Input: part model. Units: mm. Frame: model coordinates. A direction names the side the tool comes from. Give positions to 0.01 mm unless a question says otherwise; leave off trailing zeros. Write each loop counter-clockwise with the first axis right and the second up, starting at its lowest first coordinate (ties: lowest second). Pieces come first, ordered by that corner, then holes.
```python
from build123d import *

# Parameters (mm, degrees)
SKETCH1_R           = 10.16
BOSS_EXTRUDE1_DEPTH = 66.04
SKETCH2_R           = 12.7
BOSS_EXTRUDE2_DEPTH = 2.54
BOSS_EXTRUDE3_START = -2.54
SKETCH3_R           = 12.7
BOSS_EXTRUDE3_DEPTH = 2.54


with BuildPart() as part:
    # Sketch1 → Boss-Extrude1 (new, symmetric)
    with BuildSketch(Plane(origin=(0, 0, 0), x_dir=(1, 0, 0), z_dir=(0, 1, 0))):
        with Locations(Location((0, 0, 0), (0, 0, 270))):
            Circle(SKETCH1_R)
    extrude(amount=BOSS_EXTRUDE1_DEPTH, both=True)

    # Sketch2 → Boss-Extrude2 (add)
    with BuildSketch(Plane(origin=(0, 66.04, 0), x_dir=(1, 0, 0), z_dir=(0, 1, 0))):
        with Locations(Location((0, 0, 0), (0, 0, 270))):
            Circle(SKETCH2_R)
    extrude(amount=-BOSS_EXTRUDE2_DEPTH)

    # Sketch3 → Boss-Extrude3 (add)
    with BuildSketch(Plane.XZ.offset(66.04).offset(BOSS_EXTRUDE3_START)):
        with Locations(Location((0, 0, 0), (0, 0, 90))):
            Circle(SKETCH3_R)
    extrude(amount=BOSS_EXTRUDE3_DEPTH)


solid = part.part
```
Item 1: Mould query, pull axis Y, two halves, no side actions, for faces 3 (the cylindrical face through (7.7, -64.8, -10.1)), 4 (the flat face through (0, -66.04, 0)), 5 (the flat face through (0, 66.04, 0)), 6 (the flat face through (9, 63.5, -6)). Classes: +Y half, -Y half, draft (parallel to the pull), parting line (faces both ways), or undercut.
Item 2: Ray query, line 1 (Y direction, x = 1.75, z = -10.5); line 2 (Z direction, x = -0.5, y = 18). Return the intervals inside material, ascending.
Item 3: Section B-B (x = -8). Return loops of the section in (y, z), and give its area (3 significant figures).
Item 4: Set-up query: faces 1 (the flat face through (-9, -63.5, -6)), 2 (the cylindrical face through (-7.7, 64.8, -10.1)). Return all of +Z, -Z, +X, -X, +Y, -Y with unobstructed straight access to the full face (end or side cutting, diameter ignored); none if empty.
Item 5: Section C-C (y = 9.5). Return loops of the section in (x, z).
Item 6: Pin query (flat end, axial travel): pin 1 (5 mm diameter, centred on x = -2, y = -1, fed in from -Z); pin 2 (10 mm diameter, centred on y = -45, z = 2, fed in from +X); pin 3 (2 mm diameter, centred on x = -8.5, y = 14, fed in from +Z). Return the tip coordinate at first contact, or that it passes through.
Item 7: Section A-A (z = 0). Return loops of the section in (x, y), and give its area (3 significant figures).
Solved:
1. face 3: draft
1. face 4: -Y half
1. face 5: +Y half
1. face 6: undercut
2. line 1: y = -66.04 to -63.5, 63.5 to 66.04
2. line 2: z = -10.15 to 10.15
3. outline: (-66.04, -9.86) - (-63.5, -9.86) - (-63.5, -6.26) - (63.5, -6.26) - (63.5, -9.86) - (66.04, -9.86) - (66.04, 9.86) - (63.5, 9.86) - (63.5, 6.26) - (-63.5, 6.26) - (-63.5, 9.86) - (-66.04, 9.86) - close
3. area: 1,690 mm2
4. face 1: none
4. face 2: +Y, -Y
5. outline: circle Ø20.32 at (0, 0)
6. pin 1: stops at z = -10.16
6. pin 2: stops at x = 10.16
6. pin 3: stops at z = 6.85
7. outline: (-12.7, -66.04) - (12.7, -66.04) - (12.7, -63.5) - (10.16, -63.5) - (10.16, 63.5) - (12.7, 63.5) - (12.7, 66.04) - (-12.7, 66.04) - (-12.7, 63.5) - (-10.16, 63.5) - (-10.16, -63.5) - (-12.7, -63.5) - close
7. area: 2,710 mm2
